Autodesk Inventor part; units mm, degrees
ref_plane "YZ Plane" through (0, 0, 0) normal (1, 0, 0) x (0, 1, 0)
ref_plane "XZ Plane" through (0, 0, 0) normal (0, 1, 0) x (-1, 0, 0)
ref_plane "XY Plane" through (0, 0, 0) normal (0, 0, 1) x (1, 0, 0)
sketch "Sketch1" plane through (0, 0, 0) normal (0, 1, 0) x (-1, 0, 0)
  line L0 (-10.05, -1.9) -> (10.05, -1.9)
  line L1 (10.05, -1.9) -> (10.05, 1.9)
  line L2 (10.05, 1.9) -> (-10.05, 1.9)
  line L3 (-10.05, 1.9) -> (-10.05, -1.9)
  line L4 (-10.05, -1.9) -> (10.05, 1.9) construction
  line L5 (10.05, -1.9) -> (-10.05, 1.9) construction
  point P0 (0, 0)
  dimension "d0" = 3.8
  dimension "d1" = 20.1
extrude "Extrusion1" add sketch "Sketch1" along normal blind 1
fillet "Fillet1" radius 0.5 2 edges at (10.05, 0.5, 1.9) (10.05, 0.5, -1.9)
sketch "Sketch2" plane through (-10.05, 0, -1.9) normal (-1, 0, 0) x (0, 0, 1)
  line L0 (0, 0) -> (3.8, 0)
  line L1 (3.8, 0) -> (3.8, 1)
  line L2 (0, 1) -> (3.8, 1)
  line L3 (0, 0) -> (0, 1)
  line L4 (-0.6, -3.15) -> (4.4, -3.15)
  line L5 (4.4, -3.15) -> (4.4, 1.85)
  line L6 (4.4, 1.85) -> (-0.6, 1.85)
  line L7 (-0.6, 1.85) -> (-0.6, -3.15)
  line L8 (-0.6, -3.15) -> (4.4, 1.85) construction
  line L9 (4.4, -3.15) -> (-0.6, 1.85) construction
  line L10 (-2.05, -4.6) -> (5.85, -4.6) construction
  line L11 (5.85, -4.6) -> (5.85, 3.3) construction
  line L12 (5.85, 3.3) -> (-2.05, 3.3) construction
  line L13 (-2.05, 3.3) -> (-2.05, -4.6) construction
  line L14 (-2.05, -4.6) -> (5.85, 3.3) construction
  line L15 (5.85, -4.6) -> (-2.05, 3.3) construction
  point P0 (1.9, 0)
  point P1 (1.9, -0.65)
  point P2 (1.9, -0.65)
  dimension "d5" = 5
  dimension "d6" = 5
  dimension "d7" = 7.9
  dimension "d8" = 7.9
  dimension "d9" = 3.3
  dimension "d10" = 2.5
extrude "Extrusion2" add sketch "Sketch2" against normal blind 1
properties part number "Powerpole45APCBStraight" material "Stainless Steel"
CAD build for the part. Positions are in the model's coordinates, mm. A direction names the side the tool comes from. Coordinates: 2 decimals unless noted, no trailing zeros. Order: outer loops, then holes, each group sorted by start corner. A loop starts at its lowest first (then second) coordinate and runs counter-clockwise, first axis right, second up.
(1) Saw through at B-B, the plane y = 0.8. Write the cut outline in (x, z), and give its area (3 significant figures).
Solution:
outline: (-10.05, -2.5) - (-9.05, -2.5) - (-9.05, -1.9) - (9.55, -1.9) arc R0.5 ccw to (10.05, -1.4) - (10.05, 1.4) arc R0.5 ccw to (9.55, 1.9) - (-9.05, 1.9) - (-9.05, 2.5) - (-10.05, 2.5) - close
area: 77.5 mm2
(2) Saw through at A-A, the plane z = -0.55. Write the cut outline in (x, y).
Solution:
outline: (-10.05, -3.15) - (-9.05, -3.15) - (-9.05, 0) - (10.05, 0) - (10.05, 1) - (-9.05, 1) - (-9.05, 1.85) - (-10.05, 1.85) - close
(3) Saw through at C-C, the plane x = 0.75. Write the cut outline in (y, z), and give its area (3 significant figures).
Solution:
outline: (0, -1.9) - (1, -1.9) - (1, 1.9) - (0, 1.9) - close
area: 3.80 mm2
(4) Pin check, flat tips, straight feed: pin 1 Ø1.5 at (x, y) = (-5, -1) entering from +Z; pin 2 Ø3 at (x, y) = (-7, 1.5) entering from -Z; pin 3 Ø1 at (y, z) = (0, 2) entering from +X; pin 4 Ø0.8 at (x, y) = (0.5, 0.5) entering from +Z. Stop position of each tip, or through.
Solution:
pin 1: passes through
pin 2: stops at z = -1.9
pin 3: stops at x = 10.04
pin 4: stops at z = 1.9
(5) Drill centre lines: L1, parallel to Z at x = -8.5, y = 0.7; L2, parallel to Y at x = -4.5, z = 0.3; L3, parallel to X at y = -1.15, z = 0.5. Where is each one in solid material? Low to high.
Solution:
L1: z = -1.9 to 1.9
L2: y = 0 to 1
L3: x = -10.05 to -9.05
(6) Saw through at D-D, the plane z = -2.2. Write the cut outline in (x, y), and give its area (3 significant figures).
Solution:
outline: (-10.05, -3.15) - (-9.05, -3.15) - (-9.05, 1.85) - (-10.05, 1.85) - close
area: 5.00 mm2
(7) Which spindle directions (+Z, -Z, +X, -X, +Y, -Y) get a long thin tool onto all of the face, cutting with end or side? Do faces 1 (the face through (0.1, 0.5, 1.9)), 2 (the face through (1, 1, 0)), 3 (the face through (1, 0, 0)), 4 (the face through (0.4, 0.5, -1.9)). Say none if no direction does.
Solution:
face 1: +Z, +X, +Y, -Y
face 2: +Z, -Z, +X, +Y
face 3: +Z, -Z, +X, -Y
face 4: -Z, +X, +Y, -Y
